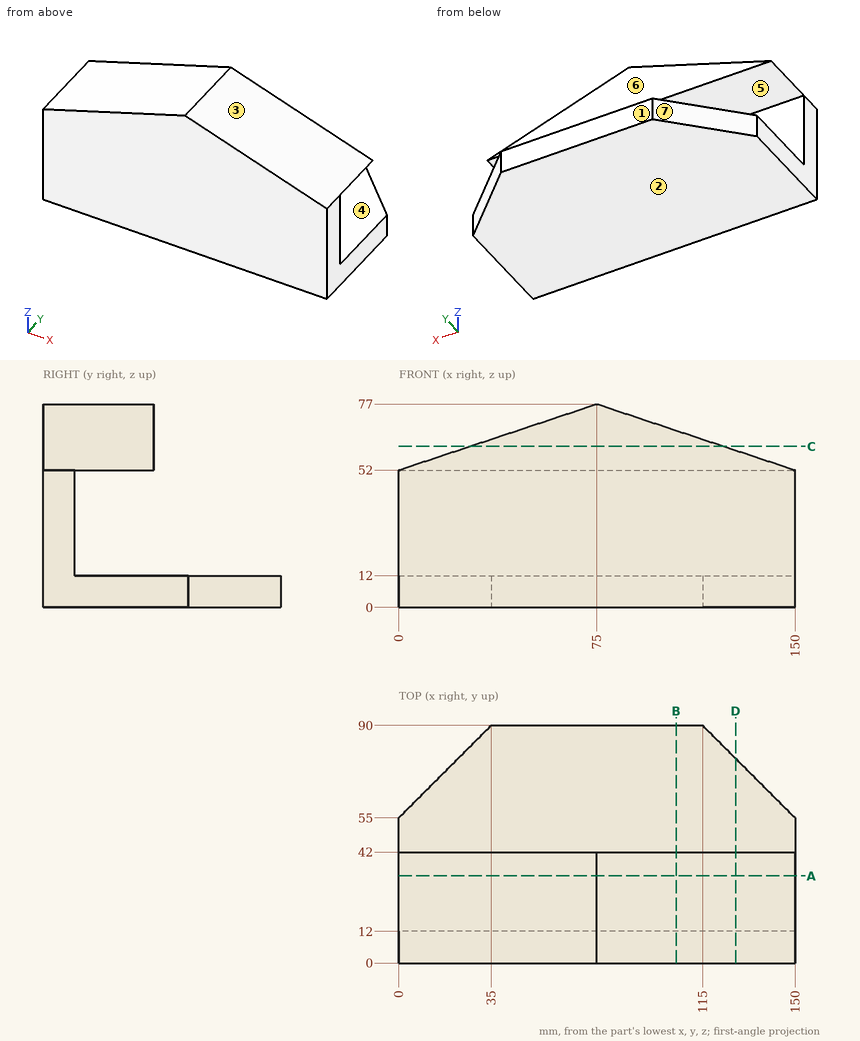
Can you work these out from the drawing? Everything is in mm from the part's minimum corner. A direction names the side the tool comes from. Coordinates: 2 decimals unless noted, no trailing zeros. Write each loop counter-clockwise with the first axis right and the second up, starting at its lowest first coordinate (ties: lowest second). Pieces come first, ordered by that corner, then holes. Notation, with made-up numbers: (65.25, 7.5) -> (69.25, 7.5) arc R17 cw to (69.25, 39.5) -> close; hole circle Ø5 at (-27.5, 84.25). An arc over 180 degrees is marked (long way). Write each question's results on one line, items separated by ' | '. Start each with the question number.
Item 1: If we section it at A-A, the plane y = 33: Write out the boundary of the cut face in (x, z).
Item 2: I'm going to push flat-ended pins straight in: P1, Ø1.5, axis at x = 118.5, y = 13, coming from the +Z side; P2, Ø5, axis at x = 114.5, y = 61, coming from the +Z side; P3, Ø10, axis at x = 111.5, y = 31.5, coming from the +Z side. Where does each tip first touch, or does it pass through?
Item 3: If we section it at D-D, the plane x = 127.5: Write out the boundary of the cut face in (y, z).
Item 4: Please list where these lines run through material, in increasing order: probe 1 along Z at (x, y) = (95, 44.5); probe 2 along Z at (x, y) = (44.5, 23).
Item 5: Thinking about a two-plate mould opening in Z: for the marked faces 1, 2, 3 and 4, which applies, released by +Z, released by -Z, zero draft, split by the parting line, or undercut?
Item 6: If we section it at C-C, the plane z = 61: Write out the boundary of the cut face in (x, y).
Item 7: If we section it at B-B, the plane x = 105: Write out the boundary of the cut face in (y, z), and give its area (3 significant figures).
Item 8: On a 3-axis mill with a long thin cutter (end or side, diameter ignored), from which of +Z, -Z, +X, -X, +Y, -Y can I reach the whole of each face in a straight line? I mean the marked faces 5, 6 and 7. Say none if no direction works.
Answer block:
1) outline: (0, 0) -> (150, 0) -> (150, 12) -> (0, 12) -> close; (0, 52) -> (150, 52) -> (75, 77) -> close
2) P1: z = 62.75 | P2: z = 12 | P3: z = 66.5
3) outline: (0, 0) -> (77.5, 0) -> (77.5, 12) -> (12, 12) -> (12, 52) -> (42, 52) -> (42, 59.5) -> (0, 59.5) -> close
4) probe 1: 0 to 12 | probe 2: 0 to 12, 52 to 66.83
5) face 1: zero draft | face 2: released by -Z | face 3: released by +Z | face 4: undercut
6) outline: (27, 0) -> (123, 0) -> (123, 42) -> (27, 42) -> close
7) outline: (0, 0) -> (90, 0) -> (90, 12) -> (12, 12) -> (12, 52) -> (42, 52) -> (42, 67) -> (0, 67) -> close | area: 2,190 mm²
8) face 5: +X, -X, +Y | face 6: +Z, +X, -X, +Y | face 7: +Z, -Z, -X, +Y
